Study the drawing (mm; zero at the part's minimum x, y, z) and answer. A direction names the side the tool comes from. Give positions to 0.01 mm unless a question says otherwise; leave off trailing zeros. Loops run counter-clockwise (first coordinate to the right, second up) from the corner with the lowest first, then second, coordinate; pieces in that order, holes last. Notation, with made-up numbers: (76.5, -30.5) -> (127.5, -30.5) arc R16 cw to (127.5, -16.5) -> close; hole circle Ø11 at (41.25, 82.5). An arc over 180 degrees is marked (long way). One line per question, with ' | ' between items. Start each with the question number.
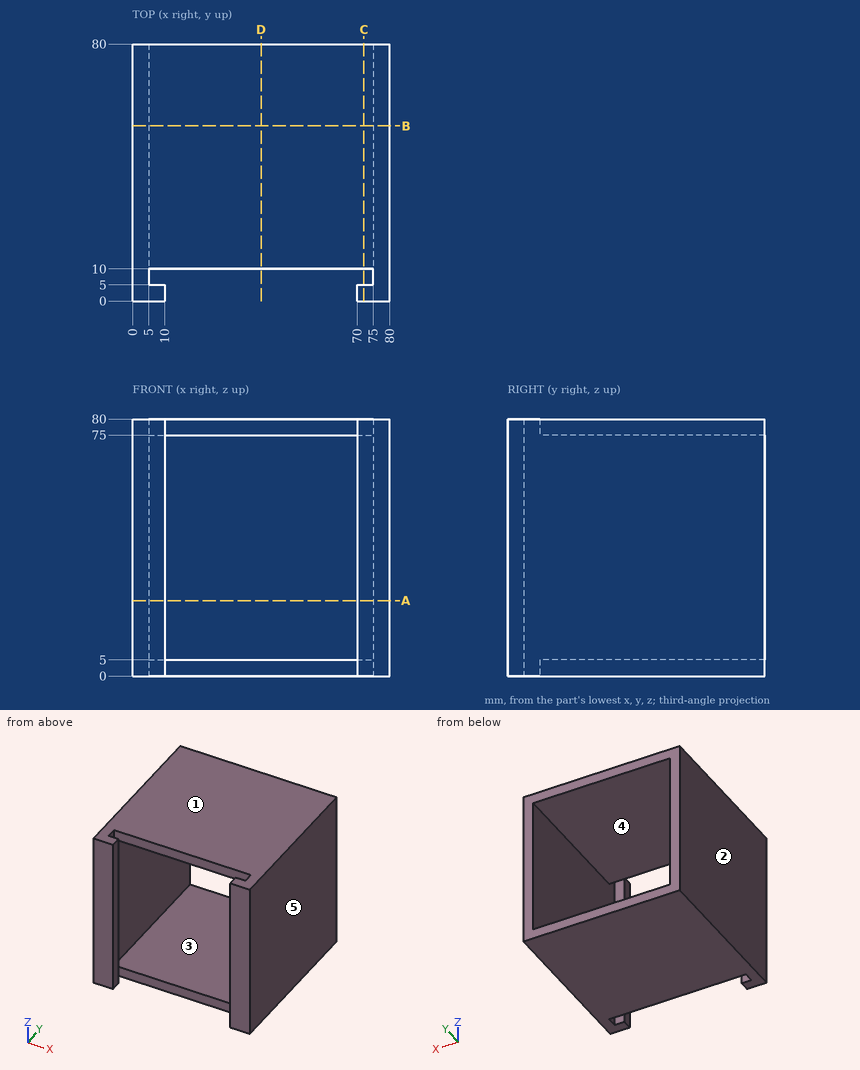
1. A straight line is drawn through the part: L1, parallel to Z at x = 63, y = 76. Find the intervals that lie inside material, in ascending order.
2. The part is cut by section A-A (z = 23.5). Write down the section's boundary in (x, y).
3. The part is cut by section C-C (x = 72). Write down the section's boundary in (y, z).
4. The part is cut by section B-B (y = 54.5). Write down the section's boundary in (x, z).
5. The part is cut by section D-D (x = 40). Write down the section's boundary in (y, z), plus the area to 3 significant figures.
6. For the marked faces 4 and 5, determine the directions among +Z, -Z, +X, -X, +Y, -Y from which every point of the face is accessible in a straight line to the end or side of a thin tool.
7. Each of these flat-tipped pins is pushed along its axis until it touches: pin 1 Ø2 at (x, z) = (68.5, 9.5) entering from -Y; pin 2 Ø1.5 at (x, z) = (34, 77.5) entering from -Y; pin 3 Ø4 at (x, z) = (8, 35) entering from +Y. Where does it stop, or does it pass through?
8. Determine the mould class of the marked faces 1, 2 and 3 for opening direction X: released by +X, released by -X, zero draft, split by the parting line, or undercut.
Check sheet entries:
1) L1: z = 0 to 5, 75 to 80
2) outline: (0, 0) -> (10, 0) -> (10, 5) -> (5, 5) -> (5, 80) -> (0, 80) -> close; (70, 0) -> (80, 0) -> (80, 80) -> (75, 80) -> (75, 5) -> (70, 5) -> close
3) outline: (0, 0) -> (5, 0) -> (5, 80) -> (0, 80) -> close; (10, 0) -> (80, 0) -> (80, 5) -> (10, 5) -> close; (10, 75) -> (80, 75) -> (80, 80) -> (10, 80) -> close
4) outline: (0, 0) -> (80, 0) -> (80, 80) -> (0, 80) -> close; hole (5, 5) -> (75, 5) -> (75, 75) -> (5, 75) -> close
5) outline: (10, 0) -> (80, 0) -> (80, 5) -> (10, 5) -> close; (10, 75) -> (80, 75) -> (80, 80) -> (10, 80) -> close | area: 700 mm^2
6) face 4: +Y | face 5: +Z, -Z, +X, +Y, -Y
7) pin 1: passes through | pin 2: stops at y = 10 | pin 3: stops at y = 5
8) face 1: zero draft | face 2: released by -X | face 3: undercut
